```python
from build123d import *

# Parameters (mm, degrees)
PAD017_DEPTH         = 16.8
PAD017_DEPTH_BACK    = 16.8
POCKET017_DEPTH      = 9.5
POCKET017_DEPTH_BACK = 9.5
CHAMFER009_SIZE      = 0.3
POCKET018_DEPTH      = 15.866909


with BuildPart() as part:
    # Sketch033 → Pad017 (new body, two sides)
    with BuildSketch(Plane.XY) as pad017_sk:
        with BuildLine():
            Line((-16.8, 10.7), (16.8, 10.7))
            Line((16.8, 10.7), (16.8, 19.183587))
            ThreePointArc((16.8, 19.183587), (0, 25.5), (-16.8, 19.183587))
            Line((-16.8, 10.7), (-16.8, 19.183587))
        make_face()
    extrude(amount=PAD017_DEPTH)
    extrude(pad017_sk.sketch, amount=-PAD017_DEPTH_BACK)

    # Sketch034 → Pocket017 (cut, two sides)
    with BuildSketch(Plane.XY) as pocket017_sk:
        with BuildLine():
            Line((-15.2, 15.466909), (15.2, 15.466909))
            Line((15.2, 15.466909), (21, 11.466909))
            Line((21, 11.466909), (23, 11.466909))
            ThreePointArc((24.265231, 8.466909), (23.680172, 9.986965), (23, 11.466909))
            Line((11, 10.5), (24.265231, 8.466909))
            Line((11, 10.5), (-11, 10.5))
            Line((-11, 10.5), (-24.265231, 8.466909))
            ThreePointArc((-23, 11.466909), (-23.680172, 9.986965), (-24.265231, 8.466909))
            Line((-21, 11.466909), (-23, 11.466909))
            Line((-15.2, 15.466909), (-21, 11.466909))
        make_face()
    extrude(amount=-POCKET017_DEPTH, mode=Mode.SUBTRACT)
    extrude(pocket017_sk.sketch, amount=POCKET017_DEPTH_BACK, mode=Mode.SUBTRACT)

    # Chamfer009
    chamfer009_edges = [part.edges().sort_by_distance(p)[0] for p in [
        (-16.8, 14.363461, 0),
        (16.8, 14.363461, 0),
    ]]
    chamfer(chamfer009_edges, length=CHAMFER009_SIZE)

    # Sketch035 → Pocket018 (cut)
    with BuildSketch(Plane.XZ):
        with BuildLine():
            Line((-4, 14.974979), (-4, 27.304979))
            Line((-4, 27.304979), (4, 27.304979))
            Line((4, 27.304979), (4, 14.974979))
            ThreePointArc((4, -14.974979), (15.5, 0), (4, 14.974979))
            Line((4, -27.304979), (4, -14.974979))
            Line((-4, -27.304979), (4, -27.304979))
            Line((-4, -14.974979), (-4, -27.304979))
            ThreePointArc((-4, 14.974979), (-15.5, 0), (-4, -14.974979))
        make_face()
    extrude(amount=-POCKET018_DEPTH, mode=Mode.SUBTRACT)


with BuildPart() as part_1:
    # Body015 placement: moved
    add(part.part.moved(Location((0, 135, 0))))


solid = part_1.part
```
Part model, mm, in its own coordinate system. A direction names the side the tool comes from. Round coordinates to 2 decimals unless told otherwise and drop trailing zeros. Write each loop counter-clockwise with the first axis right and the second up, starting at its lowest first coordinate (ties: lowest second). Pieces come first, ordered by that corner, then holes. Notation, with made-up numbers: M -19.5,-39 L 21.5,-39 A10 ccw 21.5,-28 Z; hole C 26.5,-8.5 d2. An arc over 180 degrees is marked long. Answer as CSV lines item,"result". Start each with the question number.
1) Band-saw the part on C-C (z = 11.5). List the corners of the cut face in (x, y), then the cut area to 3 significant figures.
2) Mould opens along Z. For faces 1 (the face through (15, 148, -9.5)), 2 (the face through (-14, 150.467, -8)), 3 (the face through (0, 153, -16.8)), 4 (the face through (-12, 145.7, 14)) say: +Z half, -Z half, draft (parallel to the pull), parting line (faces both ways), or undercut.
3) Band-saw the part on D-D (y = 157.5). List the corners of the cut face in (x, z).
4) Drill centre lines: L1, parallel to X at y = 150.5, z = -4; L2, parallel to Z at x = 14, y = 148.5; L3, parallel to X at y = 150.25, z = -8.5. Where is each one in solid material? Low to high.
5) Band-saw the part on B-B (x = -10). List the corners of the cut face in (y, z), then the cut area to 3 significant figures.
6) Band-saw the part on A-A (y = 147.5). List the corners of the cut face in (x, z), then the cut area to 3 significant figures.
7) Which spindle directions (+Z, -Z, +X, -X, +Y, -Y) get a long thin tool onto all of the face, cutting with end or side? Do faces 5 (the face through (-12, 145.7, -14)), 6 (the face through (4, 148, -16)), 7 (the face through (15.867, 150.007, 0.133)). Say none if no direction does.
8) Drop flat-ended pins along their axis: pin 1 (0.9 mm diameter, centred on x = -13, z = 5, fed in from -Y); pin 2 (1.5 mm diameter, centred on x = 12, z = -11.5, fed in from +Y); pin 3 (12 mm diameter, centred on x = 11.5, z = 6.5, fed in from +Y). Give the stop position or say it passes through.
Worked out:
1,outline,"M -16.8,145.7 L -10.39,145.7 L -10.39,150.87 L 10.39,150.87 L 10.39,145.7 L 16.8,145.7 L 16.8,154.18 A25.5 ccw -16.8,154.18 Z"
1,area,"323 mm²"
2,face 1,"undercut"
2,face 2,"undercut"
2,face 3,"-Z half"
2,face 4,"draft"
3,outline,"M -12,-16.8 L 12,-16.8 L 12,16.8 L -12,16.8 Z"
4,L1,"-16.8 to -14.97, 14.97 to 16.8"
4,L2,"-16.8 to -9.5, 9.5 to 16.8"
4,L3,"-16.8 to -15.51, 15.51 to 16.8"
5,outline,"M 145.7,-16.8 L 158.46,-16.8 L 158.46,16.8 L 145.7,16.8 L 145.7,11.84 L 150.87,11.84 L 150.87,-11.84 L 145.7,-11.84 Z"
5,area,"306 mm²"
6,outline,"M -16.8,-16.8 L -4,-16.8 L -4,-14.97 A15.5 cw -12.25,-9.5 L -16.8,-9.5 Z; M -16.8,9.5 L -12.25,9.5 A15.5 cw -4,14.97 L -4,16.8 L -16.8,16.8 Z; M 4,-16.8 L 16.8,-16.8 L 16.8,-9.5 L 12.25,-9.5 A15.5 cw 4,-14.97 Z; M 4,14.97 A15.5 cw 12.25,9.5 L 16.8,9.5 L 16.8,16.8 L 4,16.8 Z"
6,area,"262 mm²"
7,face 5,"+Z, -Z, +X, -X, -Y"
7,face 6,"+Z, -Z, -Y"
7,face 7,"-Y"
8,pin 1,"y = 150.87"
8,pin 2,"y = 157.88"
8,pin 3,"y = 159.9"
